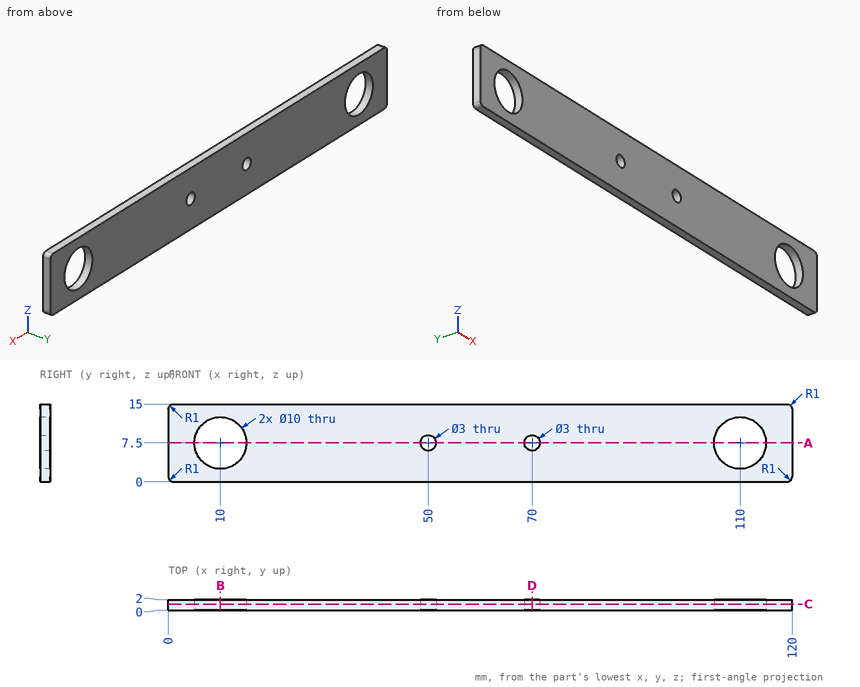
Drawing for the job (mm, zero at the part's lowest x, y, z). Coordinates: 2 decimals unless noted, no trailing zeros. Order: outer loops, then holes, each group sorted by start corner. A loop starts at its lowest first (then second) coordinate and runs counter-clockwise, first axis right, second up. Notation, with made-up numbers: (43, 42) -> (49, 42) arc R25 ccw to (49, 70) -> close; hole circle Ø11 at (-0.5, -31.75). An arc over 180 degrees is marked (long way). One line per item, written item: value.
(1) Slice it at A-A, the plane z = 7.5. List the corners of the cut face in (x, y), plus the area to 3 significant figures.
Checked values:
outline: (0, 0) -> (5, 0) -> (5, 2) -> (0, 2) -> close; (15, 0) -> (48.5, 0) -> (48.5, 2) -> (15, 2) -> close; (51.5, 0) -> (68.5, 0) -> (68.5, 2) -> (51.5, 2) -> close; (71.5, 0) -> (105, 0) -> (105, 2) -> (71.5, 2) -> close; (115, 0) -> (120, 0) -> (120, 2) -> (115, 2) -> close
area: 188 mm2
(2) Slice it at B-B, the plane x = 10. List the corners of the cut face in (y, z), plus the area to 3 significant figures.
Checked values:
outline: (0, 0) -> (2, 0) -> (2, 2.5) -> (0, 2.5) -> close; (0, 12.5) -> (2, 12.5) -> (2, 15) -> (0, 15) -> close
area: 10.0 mm2
(3) Probe line 1 (X direction, y = 0.75, z = 7.5); line 2 (Z direction, x = 70, y = 1.5); line 3 (X direction, y = 1.55, z = 11). List the from-to ranges inside material, lowest first. Write a range as [from, to].
Checked values:
line 1: [0, 5], [15, 48.5], [51.5, 68.5], [71.5, 105], [115, 120]
line 2: [0, 6], [9, 15]
line 3: [0, 6.43], [13.57, 106.43], [113.57, 120]
(4) Slice it at D-D, the plane x = 70. List the corners of the cut face in (y, z), plus the area to 3 significant figures.
Checked values:
outline: (0, 0) -> (2, 0) -> (2, 6) -> (0, 6) -> close; (0, 9) -> (2, 9) -> (2, 15) -> (0, 15) -> close
area: 24.0 mm2
(5) Slice it at C-C, the plane y = 1.2. List the corners of the cut face in (x, z), plus the area to 3 significant figures.
Checked values:
outline: (0, 1) arc R1 ccw to (1, 0) -> (119, 0) arc R1 ccw to (120, 1) -> (120, 14) arc R1 ccw to (119, 15) -> (1, 15) arc R1 ccw to (0, 14) -> close; hole circle Ø10 at (10, 7.5); hole circle Ø3 at (50, 7.5); hole circle Ø3 at (70, 7.5); hole circle Ø10 at (110, 7.5)
area: 1,630 mm2
